Autodesk Inventor part; units mm, degrees
ref_plane "YZ Plane" through (0, 0, 0) normal (1, 0, 0) x (0, 1, 0)
ref_plane "XZ Plane" through (0, 0, 0) normal (0, 1, 0) x (-1, 0, 0)
ref_plane "XY Plane" through (0, 0, 0) normal (0, 0, 1) x (1, 0, 0)
sketch "Sketch1" plane through (0, 0, 0) normal (0, 1, 0) x (-1, 0, 0)
  line L0 (0, 0) -> (70, 0)
  line L1 (70, 0) -> (70, -70)
  line L2 (70, -70) -> (0, -70)
  line L3 (0, -70) -> (0, 0)
  dimension "d0" = 70
  dimension "d1" = 70
extrude "Extrusion1" add sketch "Sketch1" along normal blind 350
sketch "Sketch2" plane through (0, 350, 0) normal (0, 1, 0) x (1, 0, 0)
  line L0 (-10, 10) -> (-60, 10)
  line L1 (-60, 10) -> (-60, 60)
  line L2 (-60, 60) -> (-10, 60)
  line L3 (-10, 60) -> (-10, 10)
  line L4 (-70, 0) -> (0, 0)
  line L5 (0, 0) -> (0, 70)
  dimension "d4" = 50
  dimension "d5" = 50
  dimension "d6" = 10
  dimension "d7" = 10
extrude "Extrusion2" cut sketch "Sketch2" against normal blind 50
chamfer "Chamfer1" distance 5 angle 45 4 edges at (-60, 350, -35) (-35, 350, -60) (-10, 350, -35) (-35, 350, -10)
sketch "Sketch3" plane through (0, 0, 0) normal (0, -1, 0) x (1, 0, 0)
  line L0 (-20, 65) -> (-50, 65)
  line L1 (-50, 65) -> (-50, -135)
  line L2 (-50, -135) -> (-20, -135)
  line L3 (-20, -135) -> (-20, 65)
  line L4 (65, -20) -> (-135, -20)
  line L5 (-135, -20) -> (-135, -50)
  line L6 (-135, -50) -> (65, -50)
  line L7 (65, -50) -> (65, -20)
  line L8 (0, 0) -> (0, -70)
  line L9 (0, -70) -> (-70, -70)
  line L10 (-70, -70) -> (-70, 0)
  point P0 (-50, -50)
  point P1 (-20, -50)
  point P2 (-20, -20)
  point P3 (-50, -20)
  dimension "d14" = 200
  dimension "d15" = 200
  dimension "d16" = 20
  dimension "d17" = 30
  dimension "d18" = 30
  dimension "d19" = 20
  dimension "d20" = 65
  dimension "d21" = 65
extrude "Extrusion3" add sketch "Sketch3" against normal blind 50 contours L3 L4 L1 L0 | L4 L8 L6 L3 | L3 L6 L1 L4 | L1 L6 L10 L4 | L3 L9 L1 L6 | L4 L7 L6 L8 | L10 L6 L5 L4 | L3 L2 L1 L9
chamfer "Chamfer2" distance 40 angle 45 4 edges at (-35, 50, 65) (-135, 50, -35) (-35, 50, -135) (65, 50, -35)
properties part number "FlipperStand"
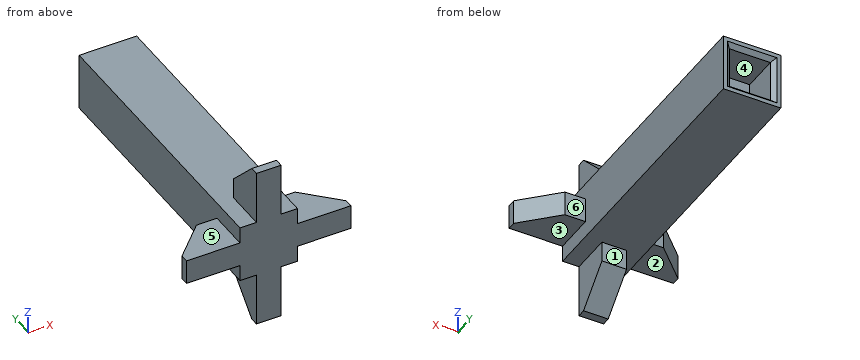
The model under review builds one solid part; all positions refer to its coordinate system, in mm. Face numbers are marked on the shaded views. A direction names the side the tool comes from. Round coordinates to 2 decimals unless told otherwise and drop trailing zeros. Loops run counter-clockwise (first coordinate to the right, second up) from the corner with the lowest first, then second, coordinate; pieces in that order, holes last. Notation, with made-up numbers: (3.5, -20.75) -> (38.5, -20.75) arc R21 cw to (38.5, 16.25) -> close; hole circle Ø9 at (76, -38). An arc over 180 degrees is marked (long way). Write item = value, one per line. Start each with the question number.
Item 1: Mouldability with a two-part tool opening along Z and no side actions: class the marked faces 4, 5 and 6 as released by +Z, released by -Z, zero draft, split by the parting line, or undercut.
Item 2: Take a section at A-A on x = -30. Give the boundary of the cut face in (y, z).
Item 3: Take a section at B-B on y = 40. Give the boundary of the cut face in (x, z).
Item 4: Take a section at D-D on z = -102. Give the boundary of the cut face in (x, y), plus the area to 3 significant figures.
Item 5: For the marked faces 1, 2 and 3, list the 3-axis set-ups (+Z, -Z, +X, -X, +Y, -Y) from which the entire face can be reached by the end or side of a thin tool; tool diameter is ignored.
Item 6: Insertion check: pin 1 (4 mm diameter, centred on x = -8, z = -17.5, fed in from +Y); pin 2 (21 mm diameter, centred on x = -21, y = 138, fed in from +Z); pin 3 (25 mm diameter, centred on x = 43.5, y = 32, fed in from -Z). Each pin has a flat end and moves straight along its axis. Give the tip position at first contact, or say it passes through.
Item 7: To check wall thickness, follow L1, parallel to Z at x = -24, y = 323; L2, parallel to Z at x = -53.5, y = 138.5. State the ranges of each line that lie inside material, in increasing order.
Item 8: Take a section at C-C on z = -40. Give the boundary of the cut face in (x, y), plus the area to 3 significant figures.
Result:
q1.face_4 = undercut
q1.face_5 = released by +Z
q1.face_6 = zero draft
q2.outline = (0, -135) -> (10, -135) -> (50, -95) -> (50, -70) -> (350, -70) -> (350, -65) -> (345, -60) -> (300, -60) -> (300, -10) -> (345, -10) -> (350, -5) -> (350, 0) -> (50, 0) -> (50, 25) -> (10, 65) -> (0, 65) -> close
q3.outline = (-105, -50) -> (-70, -50) -> (-70, -70) -> (-50, -70) -> (-50, -105) -> (-20, -105) -> (-20, -70) -> (0, -70) -> (0, -50) -> (35, -50) -> (35, -20) -> (0, -20) -> (0, 0) -> (-20, 0) -> (-20, 35) -> (-50, 35) -> (-50, 0) -> (-70, 0) -> (-70, -20) -> (-105, -20) -> close
q4.outline = (-50, 0) -> (-20, 0) -> (-20, 43) -> (-50, 43) -> close
q4.area = 1,290 mm²
q5.face_1 = -Z, +X, -X, +Y
q5.face_2 = -Z, -X, +Y, -Y
q5.face_3 = -Z, +X, +Y, -Y
q6.pin_1 = 349
q6.pin_2 = 0
q6.pin_3 = -50
q7.L1 = -70 to -60, -10 to 0
q7.L2 = -70 to 0
q8.outline = (-135, 0) -> (65, 0) -> (65, 10) -> (25, 50) -> (0, 50) -> (0, 350) -> (-5, 350) -> (-10, 345) -> (-10, 300) -> (-60, 300) -> (-60, 345) -> (-65, 350) -> (-70, 350) -> (-70, 50) -> (-95, 50) -> (-135, 10) -> close
q8.area = 26,900 mm²
